from build123d import *

# Parameters (mm, degrees)
F0_W     = 100
F0_H     = 30
F1_DEPTH = 15
F3_DEPTH = 15.001
F5_DEPTH = 30.001


with BuildPart() as f1:
    # F0 (on Top) → F1 (new body)
    with BuildSketch(Plane.XY):
        Rectangle(F0_W, F0_H)
    extrude(amount=F1_DEPTH)

    # F2 (on face) → F3 (cut, through all)
    with BuildSketch(Plane.XY.offset(15)):
        Polygon((-38.4, 4.95), (-41.7, 4.95), (-41.7, 1.65), (-45, 1.65), (-45, -1.65), (-41.7, -1.65), (-41.7, -4.95), (-38.4, -4.95), (-38.4, -1.65), (-35.1, -1.65), (-35.1, 1.65), (-38.4, 1.65), align=None)
        Polygon((-23.1, 1.65), (-23.1, -1.65), (-19.8, -1.65), (-19.8, -4.95), (-16.5, -4.95), (-16.5, -1.65), (-13.2, -1.65), (-13.2, 1.65), (-16.5, 1.65), (-16.5, 4.95), (-19.8, 4.95), (-19.8, 1.65), align=None)
        Polygon((-1.2, 1.65), (-1.2, -1.65), (2.1, -1.65), (2.1, -4.95), (5.4, -4.95), (5.4, -1.65), (8.7, -1.65), (8.7, 1.65), (5.4, 1.65), (5.4, 4.95), (2.1, 4.95), (2.1, 1.65), align=None)
        Polygon((20.7, 1.65), (20.7, -1.65), (24, -1.65), (24, -4.95), (27.3, -4.95), (27.3, -1.65), (30.6, -1.65), (30.6, 1.65), (27.3, 1.65), (27.3, 4.95), (24, 4.95), (24, 1.65), align=None)
    extrude(amount=-F3_DEPTH, mode=Mode.SUBTRACT)

    # F4 (on face) → F5 (cut, through all)
    with BuildSketch(Plane.XZ.offset(15)):
        Polygon((-27.45, 12.45), (-30.75, 12.45), (-30.75, 9.15), (-34.05, 9.15), (-34.05, 5.85), (-30.75, 5.85), (-30.75, 2.55), (-27.45, 2.55), (-27.45, 5.85), (-24.15, 5.85), (-24.15, 9.15), (-27.45, 9.15), align=None)
        Polygon((-8.85, 9.15), (-12.15, 9.15), (-12.15, 5.85), (-8.85, 5.85), (-8.85, 2.55), (-5.55, 2.55), (-5.55, 5.85), (-2.25, 5.85), (-2.25, 9.15), (-5.55, 9.15), (-5.55, 12.45), (-8.85, 12.45), align=None)
        Polygon((13.05, 9.15), (9.75, 9.15), (9.75, 5.85), (13.05, 5.85), (13.05, 2.55), (16.35, 2.55), (16.35, 5.85), (19.65, 5.85), (19.65, 9.15), (16.35, 9.15), (16.35, 12.45), (13.05, 12.45), align=None)
        Polygon((34.95, 9.15), (31.65, 9.15), (31.65, 5.85), (34.95, 5.85), (34.95, 2.55), (38.25, 2.55), (38.25, 5.85), (41.55, 5.85), (41.55, 9.15), (38.25, 9.15), (38.25, 12.45), (34.95, 12.45), align=None)
    extrude(amount=-F5_DEPTH, mode=Mode.SUBTRACT)


solid = f1.part
The model under review builds one solid part; all positions refer to its coordinate system, in mm. A direction names the side the tool comes from. Round coordinates to 2 decimals unless told otherwise and drop trailing zeros. Write each loop counter-clockwise with the first axis right and the second up, starting at its lowest first coordinate (ties: lowest second). Pieces come first, ordered by that corner, then holes. Notation, with made-up numbers: (84, 77) - (129, 77) arc R10 cw to (129, 85) - close; hole circle Ø9 at (-3.75, 65.25). An arc over 180 degrees is marked (long way). One line per item, written item: value. Start each with the question number.
1. Consider section B-B on y = -0.5. State how many separate pieces and enclosed holes the cut face has, and give its area (3 significant figures).
2. Consider section A-A on x = 25.5. Write out the cut boundary in (y, z), and give its area (4 significant figures).
3. Consider section D-D on x = -25.5. Write out the cut boundary in (y, z), and give its area (3 significant figures).
4. To check wall thickness, follow L1, parallel to X at y = -2.5, z = 12.75; L2, parallel to X at y = 10.25, z = 9; L3, parallel to Y at x = -13.5, z = 4.75. State the ranges of each line that lie inside material, in increasing order. Write a range as from..to.
5. The part is to be moulded in two halves that separate along X. For faces 3 (the face through (-45, 0, 8)), 4 (the face through (50, 0, 7)), 5 (the face through (-50, 0, 7)), say which applies: released by +X, released by -X, zero draft, split by the parting line, or undercut.
6. Machinability: for faces 1 (the face through (-21, -1.65, 8)), 2 (the face through (-27.45, 0, 11)), which of the approach directions +Z, -Z, +X, -X, +Y, -Y give a long, thin tool a straight path to every point of the face, cutting with its end or side? Answer none if there is none.
Checks:
1. separate pieces: 5
1. enclosed holes: 4
1. area: 688 mm^2
2. outline: (-15, 0) - (-4.95, 0) - (-4.95, 15) - (-15, 15) - close; (4.95, 0) - (15, 0) - (15, 15) - (4.95, 15) - close
2. area: 301.5 mm^2
3. outline: (-15, 0) - (15, 0) - (15, 5.85) - (-15, 5.85) - close; (-15, 9.15) - (15, 9.15) - (15, 15) - (-15, 15) - close
3. area: 351 mm^2
4. L1: x = -50..-41.7, -38.4..-19.8, -16.5..2.1, 5.4..24, 27.3..50
4. L2: x = -50..-34.05, -24.15..-12.15, -2.25..9.75, 19.65..31.65, 41.55..50
4. L3: y = -15..-1.65, 1.65..15
5. face 3: undercut
5. face 4: released by +X
5. face 5: released by -X
6. face 1: +Z, -Z
6. face 2: +Y, -Y
